Geometry: final body of the model. Coordinates: model frame, mm. Face numbers are marked on the shaded views. A direction names the side the tool comes from. Coordinates: 2 decimals unless noted, no trailing zeros. Order: outer loops, then holes, each group sorted by start corner. A loop starts at its lowest first (then second) coordinate and runs counter-clockwise, first axis right, second up. Notation, with made-up numbers: (57, -33) -> (90, -33) arc R24 cw to (90, -20) -> close; hole circle Ø4 at (53.5, 5). An arc over 180 degrees is marked (long way). Answer in a Markdown table with one row per item. Add a question column.
1) Section query C-C on x = -111.5. Return the cut outline in (y, z), then the cut area to 3 significant figures.
2) Section query D-D on z = 85. Return the cut outline in (x, y).
3) Ray query, line 1 (Z direction, x = 0, y = -1); line 2 (Y direction, x = 38, z = -90); line 3 (X direction, y = 15, z = 0). Return the intervals inside material, ascending. Write a range as from..to.
4) Section query A-A on y = -16.5. Return the cut outline in (x, z), then the cut area to 3 significant figures.
5) Section query B-B on z = -89.5. Return the cut outline in (x, y), then the cut area to 3 significant figures.
6) Contact query for flat-ended pins moving along their axis: P1, Ø1.5, axis at x = 83.5, y = 7.5, coming from the +Z side; P2, Ø1.5, axis at y = 11.5, z = -43, coming from the -X side; P3, Ø2, axis at x = -3, y = -0.5, coming from the +Z side. Output: stop coordinate, or through.
7) Set-up query: the marked faces 1 and 2. Return all of +Z, -Z, +X, -X, +Y, -Y with unobstructed straight access to the full face (end or side cutting, diameter ignored); none if empty.
```python
from build123d import *

# Parameters (mm, degrees)
F5_R            = 20
F6_DEPTH        = 25
F6_COPIES_COUNT = 6


# Not quite as in the source:
# - a pattern or mirror of a feature is missing from the dataset's text; its kind, count and spacing are read off the source's solid


with BuildPart() as f3:
    # F0 (on Right) → F3 (revolve)
    with BuildSketch(Plane.YZ):
        Polygon((25, 130), (0, 130), (0, 20), (20, 20), (20, 40), (6, 55), (6, 120), (25, 120), align=None)
    revolve(axis=Axis((0, 0.1935698092, 0), (0, -1, 0)))

    # F4: F3 across plane


with BuildPart() as f3_1:
    add(f3.part)
    add(f3.part.mirror(Plane.XZ))

    # F5 (on face) → F6 (cut)
    with BuildSketch(Plane.XZ.offset(6)):
        with Locations((0, 85)):
            Circle(F5_R)
    f6 = extrude(amount=-F6_DEPTH, mode=Mode.SUBTRACT)

    # F6_copies: F6 ×6 about axis
    f6_copies_axis = Axis((0, 0, 0), (0, 1, 0))
    for i in range(1, F6_COPIES_COUNT):
        add(f6.rotate(f6_copies_axis, i * 360 / F6_COPIES_COUNT), mode=Mode.SUBTRACT)


solid = f3_1.part
```
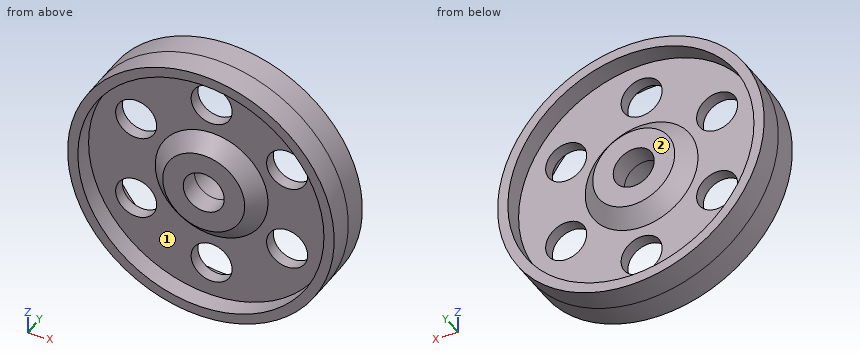
Result:
| question | item | result |
|---|---|---|
| 1 | outline | (-25, -66.84) -> (25, -66.84) -> (25, -44.36) -> (6, -44.36) -> (6, 44.36) -> (25, 44.36) -> (25, 66.84) -> (-25, 66.84) -> (-25, 44.36) -> (-6, 44.36) -> (-6, -44.36) -> (-25, -44.36) -> close |
| 1 | area | 3,310 mm2 |
| 2 | outline | (-98.36, -25) -> (-84.71, -25) -> (-84.71, -6) -> (-20, -6) -> (-20, 6) -> (-84.71, 6) -> (-84.71, 25) -> (-98.36, 25) -> close; (20, -6) -> (84.71, -6) -> (84.71, -25) -> (98.36, -25) -> (98.36, 25) -> (84.71, 25) -> (84.71, 6) -> (20, 6) -> close |
| 3 | line 1 | -130..-105, -65..-20, 20..65, 105..130 |
| 3 | line 2 | -6..6 |
| 3 | line 3 | -130..-120, -45.36..-20, 20..45.36, 120..130 |
| 4 | outline | circle Ø260 at (0, 0); circle Ø87.5 at (0, 0); hole circle Ø240 at (0, 0); hole circle Ø40 at (0, 0) |
| 4 | area | 12,600 mm2 |
| 5 | outline | (-94.29, -25) -> (-79.94, -25) -> (-79.94, -6) -> (-19.49, -6) -> (-19.49, 6) -> (-79.94, 6) -> (-79.94, 25) -> (-94.29, 25) -> close; (19.49, -6) -> (79.94, -6) -> (79.94, -25) -> (94.29, -25) -> (94.29, 25) -> (79.94, 25) -> (79.94, 6) -> (19.49, 6) -> close |
| 5 | area | 2,890 mm2 |
| 6 | P1 | z = 100.26 |
| 6 | P2 | x = -122.94 |
| 6 | P3 | z = 129.98 |
| 7 | face 1 | -Y |
| 7 | face 2 | +Y |
